Autodesk Inventor part; units mm, degrees
ref_plane "YZ Plane" through (0, 0, 0) normal (1, 0, 0) x (0, 1, 0)
ref_plane "XZ Plane" through (0, 0, 0) normal (0, 1, 0) x (-1, 0, 0)
ref_plane "XY Plane" through (0, 0, 0) normal (0, 0, 1) x (1, 0, 0)
sketch "スケッチ1" plane through (0, 0, 0) normal (0, 1, 0) x (-1, 0, 0)
  line L0 (0, 0) -> (27, 0)
  line L1 (27, 0) -> (27, -27)
  line L2 (27, -27) -> (0, -27)
  line L3 (0, -27) -> (0, 0)
  circle A0 centre (13.5, 4.5) radius 2.75
  line L4 (16.25, 4.5) -> (20.75, 4.5)
  line L5 (10.75, 4.5) -> (6.25, 4.5)
  arc A1 (16.25, 4.5) -> (20.75, 0) centre (20.75, 4.5) ccw
  arc A2 (6.25, 0) -> (10.75, 4.5) centre (6.25, 4.5) ccw
  circle A3 centre (13.5, -31.5) radius 2.75
  line L6 (10.75, -31.5) -> (6.25, -31.5)
  line L7 (16.25, -31.5) -> (20.75, -31.5)
  arc A4 (20.75, -27) -> (16.25, -31.5) centre (20.75, -31.5) ccw
  arc A5 (10.75, -31.5) -> (6.25, -27) centre (6.25, -31.5) ccw
  dimension "d0" = 27
  dimension "d1" = 27
  dimension "d11" = 5.5
  dimension "d12" = 4.5
  dimension "d13" = 4.5
  dimension "d14" = 4.5
  dimension "d15" = 5.5
  dimension "d16" = 4.5
  dimension "d17" = 4.5
  dimension "d18" = 4.5
extrude "押し出し1" add sketch "スケッチ1" along normal blind 2
sketch "スケッチ2" plane through (0, 0, 0) normal (1, 0, 0) x (0, 0, -1)
  line L0 (27, 0) -> (0, 0)
  circle A0 centre (13.5, 0) radius 13.5
  line L1 (27, 2) -> (0, 2)
  line L2 (0.149, 2) -> (26.851, 2)
  dimension "d21" = 27
extrude "押し出し2" add sketch "スケッチ2" against normal blind 27 contours L1 A0
sketch "スケッチ3" plane through (0, 2, 0) normal (0, 1, 0) x (1, 0, 0)
  arc A0 (-10.75, 31.5) -> (-16.25, 31.5) centre (-13.5, 31.5) ccw
  arc A1 (-16.25, -4.5) -> (-10.75, -4.5) centre (-13.5, -4.5) ccw
  point P0 (0, 0)
hole "穴1" at (-13.5, 2, -31.5) at (-13.5, 2, 4.5) direction (0, -1, 0) diameter 3 end through all
sketch "スケッチ4" plane through (0, 0, 0) normal (1, 0, 0) x (0, 0, -1)
  line L0 (27, 0) -> (0, 0)
  circle A0 centre (13.5, 0) radius 12
  point P0 (1.5, 0)
  point P1 (25.5, 0)
  dimension "d31" = 24
extrude "押し出し3" cut sketch "スケッチ4" against normal through all contours L0 A0 picked at (16.494, 4.567)
properties part number "daisen_moto_parts2"
Could you check a few things on this model? Use its own coordinates, in mm. A direction names the side the tool comes from. Round coordinates to 2 decimals unless told otherwise and drop trailing zeros. Loops run counter-clockwise (first coordinate to the right, second up) from the corner with the lowest first, then second, coordinate; pieces in that order, holes last.
Q1. I want a section at A-A (x = -13.5). Write out the boundary of the cut face in (y, z).
Q2. On a 3-axis mill with a long thin cutter (end or side, diameter ignored), from which of +Z, -Z, +X, -X, +Y, -Y can I reach the whole of each face in a straight line? I mean faces 5 (the flat face through (-13, 2, 2)), 6 (the flat face through (-3, 1, -27)), 7 (the flat face through (-24, 1, -27)). Say none if no direction works.
Q3. I want a section at C-C (x = -2). Write out the boundary of the cut face in (y, z).
Q4. I want a section at D-D (z = -16). Write out the boundary of the cut face in (x, y).
Q5. I want a section at B-B (y = 6). Write out the boundary of the cut face in (x, z), and give its area (3 significant figures).
Q6. Please list where these lines run through material, in increasing order: L1, parallel to X at y = 1.2, z = 4.5; L2, parallel to Z at x = -13.5, y = 1.35.
Q7. Thinking about a two-plate mould opening in X: for faces 1 (the cylindrical face through (-13.56, 0.99, -34.25)), 2 (the flat face through (-24, 1, 0)), 3 (the cylindrical face through (-12.925, 0.986, 5.886)), 4 (the cylindrical face through (-9.467, 0.986, 1.353)), which applies, pulls with the +X half, pulls with the -X half, needs draft (parallel to the pull), parting line crosses it, or undercut?
Q8. For P1, Ø1.6, axis at x = -2, y = 1, coming from the +Z side; P2, Ø6, axis at x = -4.5, y = 2.5, coming from the +Z side; P3, Ø4, axis at x = -13.5, z = 4.5, coming from the +Y side, each with a flat end and sliding along its axis, tell me the tip position at first contact or that it passes through.
Answer below:
1. outline: (0, -34.25) - (2, -34.25) - (2, -33) - (0, -33) - close; (0, -30) - (2, -30) - (2, -26.85) arc R13.5 ccw to (2, -0.15) - (2, 3) - (0, 3) - (0, -1.5) arc R12 cw to (0, -25.5) - close; (0, 6) - (2, 6) - (2, 7.25) - (0, 7.25) - close
2. face 5: +Z, +X, -X, +Y
2. face 6: -Z, +X, +Y, -Y
2. face 7: -Z, -X, +Y, -Y
3. outline: (0, -27) - (2, -27) - (2, -26.85) arc R13.5 ccw to (2, -0.15) - (2, 0) - (0, 0) - (0, -1.5) arc R12 cw to (0, -25.5) - close
4. outline: (-27, 11.74) - (0, 11.74) - (0, 13.27) - (-27, 13.27) - close
5. outline: (-27, -25.59) - (0, -25.59) - (0, -23.89) - (-27, -23.89) - close; (-27, -3.11) - (0, -3.11) - (0, -1.41) - (-27, -1.41) - close
5. area: 91.9 mm2
6. L1: x = -16.25 to -15, -12 to -10.75
6. L2: z = -34.25 to -33, -30 to -25.42, -1.58 to 3, 6 to 7.25
7. face 1: parting line crosses it
7. face 2: needs draft
7. face 3: undercut
7. face 4: pulls with the +X half
8. P1: stops at z = 0
8. P2: stops at z = 0.17
8. P3: stops at y = 2
